Build history of the part. All positions in model axes, mm. A direction names the side the tool comes from. Give positions to 0.01 mm unless a question says otherwise; leave off trailing zeros. Order: outer loops, then holes, each group sorted by start corner. A loop starts at its lowest first (then second) coordinate and runs counter-clockwise, first axis right, second up. Notation, with made-up numbers: M 23.5,83 L 80.5,83 A19 ccw 80.5,89 Z; hole C 28,44.25 d4. An arc over 180 degrees is marked long. Answer as CSV lines item,"result".
from build123d import *

# Parameters (mm, degrees)
SKETCH1_R               = 13
BOSS_EXTRUDE1_DEPTH     = 40
CHAMFER1_SIZE           = 4
SKETCH2_W               = 9.245775376
SKETCH2_H               = 49.025160165
CUT_EXTRUDE1_DEPTH      = 20
SKETCH3_W               = 9.286622431
SKETCH3_H               = 52.181973662
CUT_EXTRUDE2_DEPTH      = 20
CUT_EXTRUDE3_DEPTH      = 20
FILLET9_R               = 4
CUT_EXTRUDE4_REACH      = 50.166
SKETCH5_R               = 3.25
SKETCH6_R               = 6
BOSS_EXTRUDE2_DEPTH     = 3
CUT_EXTRUDE5_REACH      = 48.228
CUT_EXTRUDE5_END_RADIUS = 8
SKETCH7_R               = 4
CHAMFER2_SIZE           = 1


with BuildPart() as part:
    # Sketch1 → Boss-Extrude1 (new body)
    with BuildSketch(Plane(origin=(0, 0, 0), x_dir=(1, 0, 0), z_dir=(0, 1, 0))):
        with Locations(Location((0, 0, 0), (0, 0, 270))):
            Circle(SKETCH1_R)
    extrude(amount=BOSS_EXTRUDE1_DEPTH)

    # Chamfer1
    chamfer1_edges = [part.edges().sort_by_distance(p)[0] for p in [
        (0, 40, -13),
    ]]
    chamfer(chamfer1_edges, length=CHAMFER1_SIZE)

    # Sketch2 → Cut-Extrude1 (cut, symmetric)
    with BuildSketch(Plane(origin=(0, 0, 0), x_dir=(0, 0, -1), z_dir=(1, 0, 0))):
        with Locations((-16.622887688, 20.157854701)):
            Rectangle(SKETCH2_W, SKETCH2_H)
        with Locations((16.622887688, 20.157854701)):
            Rectangle(SKETCH2_W, SKETCH2_H)
    extrude(amount=CUT_EXTRUDE1_DEPTH, both=True, mode=Mode.SUBTRACT)

    # Sketch3 → Cut-Extrude2 (cut, symmetric)
    with BuildSketch(Plane.XY):
        with Locations((16.643311215, 16.67537129)):
            Rectangle(SKETCH3_W, SKETCH3_H)
        with Locations((-16.643311215, 16.67537129)):
            Rectangle(SKETCH3_W, SKETCH3_H)
    extrude(amount=CUT_EXTRUDE2_DEPTH, both=True, mode=Mode.SUBTRACT)

    # Sketch4 → Cut-Extrude3 (cut, symmetric)
    with BuildSketch(Plane.XY):
        with BuildLine():
            Line((8, 20), (8, 0))
            Line((8, 0), (-8, 0))
            Line((-8, 0), (-8, 20))
            ThreePointArc((-8, 20), (0, 28), (8, 20))
        make_face()
    extrude(amount=CUT_EXTRUDE3_DEPTH, both=True, mode=Mode.SUBTRACT)

    # Fillet9
    # the kernel refuses this fillet: 4 mm, written as the material it takes off along each edge
    with BuildSketch(Plane(origin=(0, 0, 0), x_dir=(0.9307006586833979, 0, 0.3657817435661457), z_dir=(-0.3657817435661457, 0, 0.9307006586833979))) as fillet9_piece_1:
        with BuildLine():
            CenterArc((13 - FILLET9_R, FILLET9_R), FILLET9_R, 270, 90)
            Line((13 - FILLET9_R, 0), (13, 0))
            Line((13, 0), (13, FILLET9_R))
        make_face()
    revolve(axis=Axis((0, 0, 0), (0, 1, 0)), revolution_arc=117.551393411, mode=Mode.SUBTRACT)
    with BuildSketch(Plane(origin=(0, 0, 0), x_dir=(-0.9307006586833977, 0, -0.36578174356614573), z_dir=(0.36578174356614573, 0, -0.9307006586833977))) as fillet9_piece_2:
        with BuildLine():
            CenterArc((13 - FILLET9_R, FILLET9_R), FILLET9_R, 270, 90)
            Line((13, FILLET9_R), (13, 0))
            Line((13, 0), (13 - FILLET9_R, 0))
        make_face()
    revolve(axis=Axis((0, 0, 0), (0, 1, 0)), revolution_arc=117.551393411, mode=Mode.SUBTRACT)
    with BuildSketch(Plane(origin=(12, 0, -15), x_dir=(0, 1, 0), z_dir=(0, 0, 1)), Plane(origin=(-12, 0, -15), x_dir=(1, 0, 0), z_dir=(0, 0, 1))) as fillet9_piece_3:
        with BuildLine():
            CenterArc((FILLET9_R, FILLET9_R), FILLET9_R, 180, 90)
            Line((0, FILLET9_R), (0, 0))
            Line((0, 0), (FILLET9_R, 0))
        make_face()
    extrude(amount=30, mode=Mode.SUBTRACT)
    with BuildSketch(Plane(origin=(0, 0, 0), x_dir=(-0.1061893245847588, 0, 0.9943459294150264), z_dir=(-0.9943459294150264, 0, -0.1061893245847588))) as fillet9_piece_4:
        with BuildLine():
            CenterArc((13 - FILLET9_R, FILLET9_R), FILLET9_R, 270, 90)
            Line((13 - FILLET9_R, 0), (13, 0))
            Line((13, 0), (13, FILLET9_R))
        make_face()
    revolve(axis=Axis((0, 0, 0), (0, 1, 0)), revolution_arc=117.551393411, mode=Mode.SUBTRACT)
    with BuildSketch(Plane(origin=(0, 0, 0), x_dir=(0.10618932458475924, 0, -0.9943459294150264), z_dir=(0.9943459294150264, 0, 0.10618932458475924))) as fillet9_piece_5:
        with BuildLine():
            CenterArc((13 - FILLET9_R, FILLET9_R), FILLET9_R, 270, 90)
            Line((13 - FILLET9_R, 0), (13, 0))
            Line((13, 0), (13, FILLET9_R))
        make_face()
    revolve(axis=Axis((0, 0, 0), (0, 1, 0)), revolution_arc=117.551393411, mode=Mode.SUBTRACT)

    # Cut-Extrude4: up to this face of the body (flat: up to its plane)
    cut_extrude4_end = Plane(part.part.faces().sort_by_distance((-12, 20.3320271, 0))[0])
    # Sketch5 → Cut-Extrude4 (cut, up to the picked face)
    with BuildSketch(Plane(origin=(12, 0, 0), x_dir=(0, 0, -1), z_dir=(1, 0, 0)), mode=Mode.PRIVATE) as cut_extrude4_sk1:
        with Locations(Location((0, 10, 0), (0, 0, 90))):
            Circle(SKETCH5_R)
    cut_extrude4_tool1 = split(extrude(cut_extrude4_sk1.sketch, amount=-CUT_EXTRUDE4_REACH, mode=Mode.PRIVATE), bisect_by=cut_extrude4_end, keep=Keep.BOTH, mode=Mode.PRIVATE)
    add(cut_extrude4_tool1.solids().sort_by(Axis((12, 10, 0), (-1, 0, 0)))[0], mode=Mode.SUBTRACT)

    # Sketch6 → Boss-Extrude2 (add)
    with BuildSketch(Plane(origin=(0, 40, 0), x_dir=(1, 0, 0), z_dir=(0, 1, 0))):
        with Locations(Location((0, 0, 0), (0, 0, 270))):
            Circle(SKETCH6_R)
    extrude(amount=BOSS_EXTRUDE2_DEPTH)

    # Cut-Extrude5: up to this cylinder (the profile starts outside it)
    cut_extrude5_end = Plane(origin=(0, 20, 0), z_dir=(0, 0, 1)) * Cylinder(CUT_EXTRUDE5_END_RADIUS, 113.456, mode=Mode.PRIVATE)
    # Sketch7 → Cut-Extrude5 (cut, up to the surface)
    with BuildSketch(Plane(origin=(0, 43, 0), x_dir=(1, 0, 0), z_dir=(0, 1, 0)), mode=Mode.PRIVATE) as cut_extrude5_sk1:
        with Locations(Location((0, 0, 0), (0, 0, 270))):
            Circle(SKETCH7_R)
    cut_extrude5_tool1 = extrude(cut_extrude5_sk1.sketch, amount=-CUT_EXTRUDE5_REACH, mode=Mode.PRIVATE) - cut_extrude5_end
    add(cut_extrude5_tool1.solids().sort_by_distance((0, 43, 0))[0], mode=Mode.SUBTRACT)

    # Chamfer2
    chamfer2_edges = [part.edges().sort_by_distance(p)[0] for p in [
        (0, 43, -6),
    ]]
    chamfer(chamfer2_edges, length=CHAMFER2_SIZE)


solid = part.part
Item 1: Band-saw the part on C-C (z = 0). Give the cut face in (x, y), and give its area (3 significant figures).
Geometry says:
outline,"M -12,4 A4 ccw -8,0 L -8,6.75 L -12,6.75 Z; M -12,13.25 L -8,13.25 L -8,20 A8 cw -4,26.93 L -4,43 L -5,43 L -6,42 L -6,40 L -9,40 L -12,37 Z; M 4,26.93 A8 cw 8,20 L 8,13.25 L 12,13.25 L 12,37 L 9,40 L 6,40 L 6,42 L 5,43 L 4,43 Z; M 8,0 A4 ccw 12,4 L 12,6.75 L 8,6.75 Z"
area,"384 mm2"
Item 2: Band-saw the part on B-B (x = 0). Give the cut face in (y, z).
Geometry says:
outline,"M 28,-12 L 37,-12 L 40,-9 L 40,-6 L 42,-6 L 43,-5 L 43,-4 L 28,-4 Z; M 28,4 L 43,4 L 43,5 L 42,6 L 40,6 L 40,9 L 37,12 L 28,12 Z"
Item 3: Probe line 1 along Z through (x, y) = (0, 33.25); line 2 along X through (y, z) = (9, 3.75); line 3 along Z through (x, y) = (-10.55, 10). List the from-to ranges inside material, lowest first. Write a range as from..to.
Geometry says:
line 1,"z = -12..-4, 4..12"
line 2,"x = -12..-8, 8..12"
line 3,"z = -7.6..-3.25, 3.25..7.6"
Item 4: Drop flat-ended pins along their axis: pin 1 (1 mm diameter, centred on x = -5, z = -7, fed in from -Y); pin 2 (2 mm diameter, centred on x = -9.5, z = -8.5, fed in from +Y); pin 3 (4 mm diameter, centred on y = 10, z = 0, fed in from +X); pin 4 (9 mm diameter, centred on x = 0, z = 0, fed in from -Y). Give the stop position or say it passes through.
Geometry says:
pin 1,"stops at y = 25.81"
pin 2,"stops at y = 37.25"
pin 3,"passes through"
pin 4,"stops at y = 26.61"
Item 5: Band-saw the part on A-A (y = 10). Give the cut face in (x, z).
Geometry says:
outline,"M -12,-5 A13 ccw -8,-10.25 L -8,-3.25 L -12,-3.25 Z; M -12,3.25 L -8,3.25 L -8,10.25 A13 ccw -12,5 Z; M 8,-10.25 A13 ccw 12,-5 L 12,-3.25 L 8,-3.25 Z; M 8,3.25 L 12,3.25 L 12,5 A13 ccw 8,10.25 Z"
Item 6: 3-axis set-ups, long thin cutter, end or side, ignore diameter. For faces 4 (the flat face through (-8, 14, 0)), 5 (the flat face through (-6, 40, 2)), 6 (the cylindrical face through (10, 19.776, -8.306)): which of +Z, -Z, +X, -X, +Y, -Y reach the whole face in a straight line?
Geometry says:
face 4,"+Z, -Z, -Y"
face 5,"+Y"
face 6,"-Z, +X, +Y, -Y"
Item 7: Pull direction Z, two halves, no side cores. Call faces 1 (the cylindrical face through (-9.972, 6.753, 0.143)), 2 (the cylindrical face through (9.909, 19.776, 8.415)), 3 (the flat face through (-12, 20, 0)): released by +Z, released by -Z, zero draft, split by the parting line, or undercut.
Geometry says:
face 1,"undercut"
face 2,"released by +Z"
face 3,"zero draft"
